Autodesk Inventor part; units mm, degrees
ref_plane "YZ Plane" through (0, 0, 0) normal (1, 0, 0) x (0, 1, 0)
ref_plane "XZ Plane" through (0, 0, 0) normal (0, 1, 0) x (-1, 0, 0)
ref_plane "XY Plane" through (0, 0, 0) normal (0, 0, 1) x (1, 0, 0)
sketch "Sketch1" plane through (0, 0, 0) normal (0, 1, 0) x (-1, 0, 0)
  circle A0 centre (0, 0) radius 3.175
  dimension "d2" = 6.35
extrude "Extrusion1" add sketch "Sketch1" along normal blind 44.45
thread "Thread1"
sketch "Sketch2" plane through (0, 44.45, 0) normal (0, 1, 0) x (1, 0, 0)
  circle A0 centre (0, 0) radius 4.7625
  dimension "d7" = 9.525
extrude "Extrusion2" add sketch "Sketch2" along normal blind 6.35
sketch "Sketch3" plane through (0, 50.8, 0) normal (0, 1, 0) x (1, 0, 0)
  line L0 (2.719, 2.4592) -> (3.4893, -1.1251)
  line L1 (3.4893, -1.1251) -> (0.7703, -3.5843)
  line L2 (0.7703, -3.5843) -> (-2.719, -2.4592)
  line L3 (-2.719, -2.4592) -> (-3.4893, 1.1251)
  line L4 (-3.4893, 1.1251) -> (-0.7703, 3.5843)
  line L5 (-0.7703, 3.5843) -> (2.719, 2.4592)
  point P0 (0, 0)
  point P1 (0, 0)
  dimension "d10" = 6.35
extrude "Extrusion3" cut sketch "Sketch3" against normal blind 4.318
properties part number "qtr20_75"
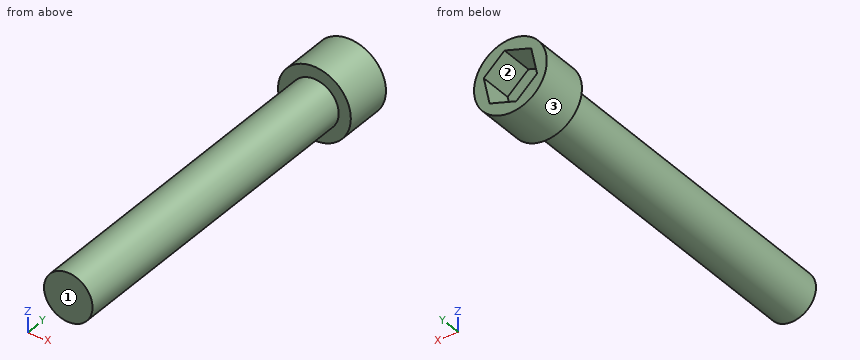
For this review, take the finished solid that the model builds, in its own axes (mm). Face numbers are marked on the shaded views. Give positions to 0.01 mm unless a question says otherwise; leave off trailing zeros. Loops run counter-clockwise (first coordinate to the right, second up) from the corner with the lowest first, then second, coordinate; pieces in that order, holes last.
Item 1: Draft analysis for pull direction Z (two halves, no side actions). For the marked faces 1, 2 and 3, state which applies: +Z half, -Z half, draft (parallel to the pull), parting line (faces both ways), or undercut.
Item 2: Insertion check: pin 1 (5 mm diameter, centred on x = 1, z = 3, fed in from -Y); pin 2 (4 mm diameter, centred on y = 8.5, z = 0.5, fed in from +X) (3 decimals). Each pin has a flat end and moves straight along its axis. Give the tip position at first contact, or say it passes through.
Item 3: For line 1 along X through (y, z) = (48.5, 0); line 2 along Y through (x, z) = (3.5, 2.75); line 3 along Z through (x, y) = (-3.25, 45), list the stretches that pass through material, from the lowest coordinate up.
Item 4: Take a section at C-C, the plane y = 28. State the section outline as (x, z) points (3 decimals).
Item 5: Take a section at D-D, the plane x = 4. State the section outline as (y, z) points.
Calculated:
1. face 1: draft
1. face 2: undercut
1. face 3: parting line
2. pin 1: stops at y = 0
2. pin 2: stops at x = 3.175
3. line 1: x = -4.76 to -3.25, 3.25 to 4.76
3. line 2: y = 44.45 to 50.8
3. line 3: z = -3.48 to 3.48
4. outline: circle Ø6.35 at (0, 0)
5. outline: (44.45, -2.58) - (50.8, -2.58) - (50.8, 2.58) - (44.45, 2.58) - close
